```python
from build123d import *

# Parameters (mm, degrees)
BASE_FLANGE1_DEPTH = 0.6
CUT_EXTRUDE1_DEPTH = 10
EDGE_FLANGE1_DEPTH = 15.014611851
CUT_EXTRUDE2_DEPTH = 10
SKETCH11_R         = 3.1
CUT_EXTRUDE3_DEPTH = 10
EDGE_FLANGE2_DEPTH = 10.6
CUT_EXTRUDE4_DEPTH = 10
CUT_EXTRUDE5_DEPTH = 10


# Sheet-metal steps are written as plain solids
with BuildPart() as part:
    # Sketch1 → Base-Flange1 (new body)
    with BuildSketch(Plane(origin=(0, 0, 0), x_dir=(1, 0, 0), z_dir=(0, 1, 0))):
        with BuildLine():
            Line((-8.474188988, 5), (6.540422863, 5))
            Line((6.540422863, 5), (6.540422863, -5))
            Line((6.540422863, -5), (-3.474188988, -5))
            ThreePointArc((-3.474188988, -5), (-7.009722894, -3.535533906), (-8.474188988, 0))
            Line((-8.474188988, 0), (-8.474188988, 5))
        make_face()
    extrude(amount=-BASE_FLANGE1_DEPTH)

    # Sketch6 → Cut-Extrude1 (cut)
    with BuildSketch(Plane(origin=(0, 0, 0), x_dir=(1, 0, 0), z_dir=(0, 1, 0))):
        with BuildLine():
            Line((6.540422863, -2.1), (-3.459577137, -2.1))
            ThreePointArc((-3.459577137, -2.1), (-5.559577137, 0), (-3.459577137, 2.1))
            Line((-3.459577137, 2.1), (6.540422863, 2.1))
            Line((6.540422863, 2.1), (6.540422863, -2.1))
        make_face()
    extrude(amount=-CUT_EXTRUDE1_DEPTH, mode=Mode.SUBTRACT)

    # Edge-Flange1 section (across the edge) → Edge-Flange1 (add)
    with BuildSketch(Plane(origin=(6.540422863, 0, -5.6), x_dir=(0, 0, 1), z_dir=(-1, 0, 0))):
        with BuildLine():
            Line((-0.6, 0.6), (-0.6, 11.2))
            Line((-0.6, 11.2), (0, 11.2))
            Line((0, 11.2), (0, 0.6))
            ThreePointArc((0, 0.6), (0.175735931, 0.175735931), (0.6, 0))
            Line((0.6, 0), (0.6, -0.6))
            ThreePointArc((0.6, -0.6), (-0.248528137, -0.248528137), (-0.6, 0.6))
        make_face()
    extrude(amount=EDGE_FLANGE1_DEPTH)

    # Sketch10 → Cut-Extrude2 (cut)
    with BuildSketch(Plane.XY.offset(-5.6)):
        with BuildLine():
            Line((-8.474188988, 6.2), (-8.474188988, 11.2))
            Line((-8.474188988, 11.2), (-3.474188988, 11.2))
            ThreePointArc((-3.474188988, 11.2), (-7.009722894, 9.735533906), (-8.474188988, 6.2))
        make_face()
    extrude(amount=-CUT_EXTRUDE2_DEPTH, mode=Mode.SUBTRACT)

    # Sketch11 → Cut-Extrude3 (cut)
    with BuildSketch(Plane.XY.offset(-5.6)):
        with Locations((-3.459577137, 4.4)):
            Circle(SKETCH11_R)
    extrude(amount=-CUT_EXTRUDE3_DEPTH, mode=Mode.SUBTRACT)

    # Edge-Flange2 section (across the edge) → Edge-Flange2 (add)
    with BuildSketch(Plane(origin=(6.712470095, 11.2, -6.2), x_dir=(-0.5299192642332, 0, -0.8480480961564292), z_dir=(0, -1, 0))):
        with BuildLine():
            Line((-0.6, 0.172047231), (-0.6, 23.827952769))
            Line((-0.6, 23.827952769), (0, 23.827952769))
            Line((0, 23.827952769), (0, 0.172047231))
            ThreePointArc((0, 0.172047231), (0.023242982, 0.006664818), (0.091171142, -0.145904327))
            Line((0.091171142, -0.145904327), (-0.417657715, -0.463855886))
            ThreePointArc((-0.417657715, -0.463855886), (-0.553514035, -0.158717596), (-0.6, 0.172047231))
        make_face()
    extrude(amount=EDGE_FLANGE2_DEPTH)

    # Sketch17 → Cut-Extrude4 (cut)
    with BuildSketch(Plane(origin=(-0.583351544, 0, -0.933557619), x_dir=(0.848048096156429, 0, -0.5299192642332), z_dir=(0.5299192642332001, 0, 0.8480480961564291))):
        with BuildLine():
            Line((14.714141037, 8.7), (27.214141037, 8.7))
            ThreePointArc((27.214141037, 8.7), (30.014141037, 5.9), (27.214141037, 3.1))
            Line((27.214141037, 3.1), (14.714141037, 3.1))
            ThreePointArc((14.714141037, 3.1), (11.914141037, 5.9), (14.714141037, 8.7))
        make_face()
        with BuildLine():
            Line((32.805949691, 11.2), (32.805949691, 0.6))
            Line((32.805949691, 0.6), (27.205949691, 0.6))
            ThreePointArc((27.205949691, 0.6), (31.058221748, 2.135519713), (32.797908203, 5.9))
            ThreePointArc((32.797908203, 5.9), (31.058221748, 9.664480287), (27.205949691, 11.2))
            Line((27.205949691, 11.2), (32.805949691, 11.2))
        make_face()
    extrude(amount=-CUT_EXTRUDE4_DEPTH, mode=Mode.SUBTRACT)

    # Sketch19 → Cut-Extrude5 (cut)
    with BuildSketch(Plane(origin=(-0.583351544, 0, -0.933557619), x_dir=(0.8480480961564292, 0, -0.5299192642331998), z_dir=(0.5299192642331998, 0, 0.8480480961564292))):
        with BuildLine():
            Line((32.733155133, 5.3), (29.949099903, 5.3))
            ThreePointArc((29.949099903, 5.3), (30.014141037, 5.9), (29.949099903, 6.5))
            Line((29.949099903, 6.5), (32.733155133, 6.5))
            ThreePointArc((32.733155133, 6.5), (32.809148381, 5.9), (32.733155133, 5.3))
        make_face()
    extrude(amount=-CUT_EXTRUDE5_DEPTH, mode=Mode.SUBTRACT)


solid = part.part
```
Work out the finished part from the listing and answer in its coordinate system (mm). A direction names the side the tool comes from. Give positions to 0.01 mm unless a question says otherwise; leave off trailing zeros. Loops run counter-clockwise (first coordinate to the right, second up) from the corner with the lowest first, then second, coordinate; pieces in that order, holes last. Notation, with made-up numbers: (0.25, 54.25) - (48.25, 54.25) arc R22 ccw to (48.25, 84.25) - close; hole circle Ø10 at (76, 1). An arc over 180 degrees is marked (long way). Use CSV: the item, a comma, the result in double quotes. Start each with the question number.
(1) Find section B-B, the plane z = -14. Determine the outline of the cut face in (x, y), plus the area to 3 significant figures.
(2) Find section A-A, the plane x = 0.5. Determine the outline of the cut face in (y, z).
(3) Find the intervals of material crossed by L1, parallel to Z at x = 2, y = 5.75; L2, parallel to Y at x = 2, z = -4.5; L3, parallel to Z at x = 14, y = 10, in increasing order.
(4) Find section D-D, the plane y = 4.4. Determine the outline of the cut face in (x, z), plus the area to 3 significant figures.
(5) Each of these flat-tipped pins is pushed along its axis until it touches: pin 1 (2 mm diameter, centred on y = 8.5, z = -13.5, fed in from -X); pin 2 (2 mm diameter, centred on x = 25.5, z = -18, fed in from -Y); pin 3 (1.6 mm diameter, centred on x = 26, z = -17.5, fed in from +Y); pin 4 (5 mm diameter, centred on x = -3.46, y = 4.4, fed in from +Z). Where does it stop, or does it pass through?
(6) Find section C-C, the plane y = 2.25. Determine the outline of the cut face in (x, z) (3 decimals), plus the area to 3 significant figures.
(7) Determine the mould class of faces 4 (the face through (23.845, 3.735, -16.547)), 5 (the face through (-0.9, 0, -2.3)), 6 (the face through (1, 6, -6.2)) for opening direction Y: released by +Y, released by -Y, zero draft, split by the parting line, or undercut.
(8) A tool of negligible diameter and unlimited length cuts with its end or side. For faces 1 (the face through (26, 6.5, -18)), 2 (the face through (17, 9.51, -12.63)), 3 (the face through (6.54, -0.3, -4.1)), from which of +Z, -Z, +X, -X, +Y, -Y can it reach the whole face along a straight path? Write none if from no direction.
Results found:
1,outline,"(19.2, 0.6) - (20.33, 0.6) - (20.33, 3.1) - (19.2, 3.1) - close; (19.2, 8.7) - (20.33, 8.7) - (20.33, 11.2) - (19.2, 11.2) - close"
1,area,"5.66 mm^2"
2,outline,"(-0.6, -5) arc R1.2 ccw to (0.6, -6.2) - (11.2, -6.2) - (11.2, -5.6) - (0.6, -5.6) arc R0.6 cw to (0, -5) - (0, -2.1) - (-0.6, -2.1) - close; (-0.6, 2.1) - (0, 2.1) - (0, 5) - (-0.6, 5) - close"
3,L1,"-6.2 to -5.6"
3,L2,"-0.6 to 0"
3,L3,"-10.75 to -10.05"
4,outline,"(-8.47, -6.2) - (-6.56, -6.2) - (-6.56, -5.6) - (-8.47, -5.6) - close; (-0.36, -6.2) - (6.54, -6.2) arc R0.6 cw to (6.86, -6.29) - (9.57, -7.99) - (9.89, -7.48) - (7.18, -5.78) arc R1.2 ccw to (6.54, -5.6) - (-0.36, -5.6) - close; (24.18, -17.12) - (26.67, -18.67) - (26.99, -18.16) - (24.5, -16.61) - close"
4,area,"9.27 mm^2"
5,pin 1,"x = 16.83"
5,pin 2,"y = 1.45"
5,pin 3,"y = 10.11"
5,pin 4,"through"
6,outline,"(-8.474, -6.2) - (-5.693, -6.2) - (-5.693, -5.6) - (-8.474, -5.6) - close; (-1.226, -6.2) - (6.54, -6.2) arc R0.6 cw to (6.858, -6.291) - (25.537, -17.963) - (25.855, -17.454) - (7.176, -5.782) arc R1.2 ccw to (6.54, -5.6) - (-1.226, -5.6) - close"
6,area,"19.8 mm^2"
7,face 4,"undercut"
7,face 5,"released by +Y"
7,face 6,"zero draft"
8,face 1,"+Z, -Z, +X, -X"
8,face 2,"-Z, -X, +Y, -Y"
8,face 3,"+Z, -Z, +X, -Y"
